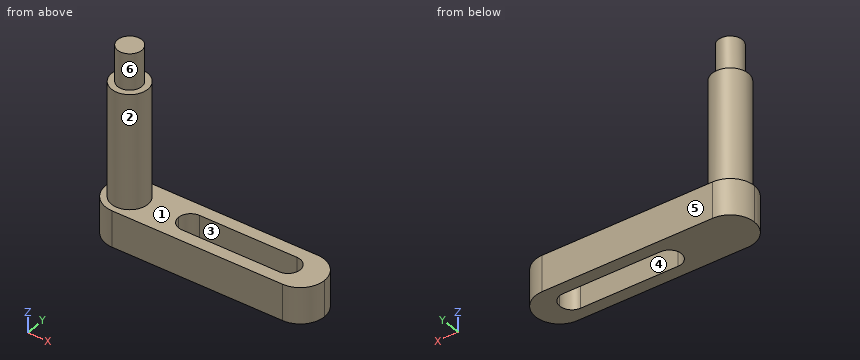
from build123d import *

# Parameters (mm, degrees)
F1_DEPTH = 6
F2_R     = 3
F3_DEPTH = 19
F4_R     = 2
F5_DEPTH = 6


with BuildPart() as f1:
    # F0 (on Top) → F1 (new body)
    with BuildSketch(Plane.XY):
        with BuildLine():
            Line((-28.736944, 4), (-56.736944, 4))
            ThreePointArc((-56.736944, 4), (-59.565371, 2.828427), (-60.736944, 0))
            ThreePointArc((-60.736944, 0), (-59.565371, -2.828427), (-56.736944, -4))
            Line((-56.736944, -4), (-28.736944, -4))
            ThreePointArc((-28.736944, -4), (-25.908517, -2.828427), (-24.736944, 0))
            ThreePointArc((-24.736944, 0), (-25.908517, 2.828427), (-28.736944, 4))
        make_face()
        with BuildLine():
            ThreePointArc((-48.736944, 0), (-48.151158, 1.414214), (-46.736944, 2))
            Line((-46.736944, 2), (-30.736944, 2))
            ThreePointArc((-30.736944, 2), (-29.32273, 1.414214), (-28.736944, 0))
            ThreePointArc((-28.736944, 0), (-29.32273, -1.414214), (-30.736944, -2))
            Line((-30.736944, -2), (-46.736944, -2))
            ThreePointArc((-46.736944, -2), (-48.151158, -1.414214), (-48.736944, 0))
        make_face(mode=Mode.SUBTRACT)
    extrude(amount=F1_DEPTH)

    # F2 (on face) → F3 (join)
    with BuildSketch(Plane.XY.offset(6)):
        with Locations((-56.736944, 0)):
            Circle(F2_R)
    extrude(amount=F3_DEPTH)

    # F4 (on face) → F5 (join)
    with BuildSketch(Plane.XY.offset(25)):
        with Locations((-56.736944, 0)):
            Circle(F4_R)
    extrude(amount=F5_DEPTH)


solid = f1.part
The listing builds one solid part. Answer for the finished solid, in the listing's coordinates (mm). Face numbers are marked on the shaded views. A direction names the side the tool comes from. Round coordinates to 2 decimals unless told otherwise and drop trailing zeros. Order: outer loops, then holes, each group sorted by start corner. A loop starts at its lowest first (then second) coordinate and runs counter-clockwise, first axis right, second up. Notation, with made-up numbers: (-30.75, -20) -> (-12.75, -20) arc R28 cw to (-12.75, 8) -> close; hole circle Ø9 at (-22, -11.5). An arc over 180 degrees is marked (long way). Write each question's results on one line, items separated by ' | '. Start each with the question number.
Q1. Find section A-A (x = -36.5). Determine the outline of the cut face in (y, z), then the cut area to 3 significant figures.
Q2. Straight lines are drawn through the part: probe 1 along Y at (x, z) = (-37, 2); probe 2 along Z at (x, y) = (-30, -2.5); probe 3 along Z at (x, y) = (-55, 2). For each, find the intervals that lie inside material, in ascending order. Write a range as from..to.
Q3. Which of the six approach directions +Z, -Z, +X, -X, +Y, -Y give full straight-line access (tool end or side, diameter ignored) to the marked faces 4, 5 and 6?
Q4. Find section B-B (z = 3.5). Determine the outline of the cut face in (x, y).
Q5. The mould has two halves that part along X. Classify the marked faces 1, 2 and 3: pulls with the +X half, pulls with the -X half, needs draft (parallel to the pull), parting line crosses it, or undercut.
Q6. Each of these flat-tipped pins is pushed along its axis until it touches: pin 1 (4 mm diameter, centred on y = -2.5, z = 15.5, fed in from +X); pin 2 (1 mm diameter, centred on y = -0.5, z = 19, fed in from -X); pin 3 (2.5 mm diameter, centred on x = -43.5, y = -1, fed in from +Z). Where does it stop, or does it pass through?
Q7. Find section C-C (y = 0.5). Determine the outline of the cut face in (x, z), then the cut area to 3 significant figures.
Q8. Find section D-D (z = 20). Determine the outline of the cut face in (x, y).
Worked answers:
1) outline: (-4, 0) -> (-2, 0) -> (-2, 6) -> (-4, 6) -> close; (2, 0) -> (4, 0) -> (4, 6) -> (2, 6) -> close | area: 24.0 mm2
2) probe 1: y = -4..-2, 2..4 | probe 2: z = 0..6 | probe 3: z = 0..25
3) face 4: +Z, -Z | face 5: +Z, -Z, +X, -X, +Y | face 6: +Z
4) outline: (-56.74, -4) -> (-28.74, -4) arc R4 ccw to (-28.74, 4) -> (-56.74, 4) arc R4 ccw to start; hole (-48.74, 0) arc R2 ccw to (-46.74, -2) -> (-30.74, -2) arc R2 ccw to (-28.74, 0) arc R2 ccw to (-30.74, 2) -> (-46.74, 2) arc R2 ccw to start
5) face 1: needs draft | face 2: parting line crosses it | face 3: undercut
6) pin 1: stops at x = -53.78 | pin 2: stops at x = -59.74 | pin 3: stops at z = 6
7) outline: (-60.71, 0) -> (-48.67, 0) -> (-48.67, 6) -> (-53.78, 6) -> (-53.78, 25) -> (-54.8, 25) -> (-54.8, 31) -> (-58.67, 31) -> (-58.67, 25) -> (-59.69, 25) -> (-59.69, 6) -> (-60.71, 6) -> close; (-28.8, 0) -> (-24.77, 0) -> (-24.77, 6) -> (-28.8, 6) -> close | area: 232 mm2
8) outline: circle Ø6 at (-56.74, 0)
